from build123d import *

# Parameters (mm, degrees)
BOSS_EXTRUDE2_DEPTH                                 = 22
SKETCH6_R                                           = 35
CUT_EXTRUDE2_DEPTH                                  = 18
CHAMFER2_SIZE                                       = 2
CIRPATTERN2_COUNT                                   = 6
M8X1_0_TAPPED_HOLE1_D                               = 7
M8X1_0_TAPPED_HOLE1_DEPTH                           = 15
M8X1_0_TAPPED_HOLE1_CSINK_D                         = 8.05
M8X1_0_TAPPED_HOLE1_CSINK_ANGLE                     = 90
M8X1_0_TAPPED_HOLE1_TIP                             = 2.103012167
CSK_FOR_M8_COUNTERSUNK_FLAT_HEAD_SCREW1_D           = 6
CSK_FOR_M8_COUNTERSUNK_FLAT_HEAD_SCREW1_DEPTH       = 20
CSK_FOR_M8_COUNTERSUNK_FLAT_HEAD_SCREW1_CSINK_D     = 8
CSK_FOR_M8_COUNTERSUNK_FLAT_HEAD_SCREW1_CSINK_ANGLE = 90
CSK_FOR_M8_COUNTERSUNK_FLAT_HEAD_SCREW1_TIP         = 1.802581857
SKETCH15_R                                          = 14
BOSS_EXTRUDE3_DEPTH                                 = 7
FILLET1_R                                           = 4
SKETCH16_R                                          = 10
CUT_EXTRUDE3_DEPTH                                  = 30


with BuildPart() as part:
    # Sketch1 → Boss-Extrude2 (new body)
    with BuildSketch(Plane.XY):
        with BuildLine():
            Line((0, 47.5), (38, 47.5))
            Line((38, 47.5), (38, 28.5))
            ThreePointArc((38, 28.5), (47.349517724, -3.777985082), (33, -34.165040612))
            Line((33, -34.165040612), (33, -45.5))
            ThreePointArc((33, -45.5), (34.171572875, -48.328427125), (37, -49.5))
            Line((37, -49.5), (50, -49.5))
            Line((50, -49.5), (50, -59.5))
            Line((50, -59.5), (-50, -59.5))
            Line((-50, -59.5), (-50, -49.5))
            Line((-50, -49.5), (-37, -49.5))
            ThreePointArc((-37, -49.5), (-34.171572875, -48.328427125), (-33, -45.5))
            Line((-33, -45.5), (-33, -34.165040612))
            ThreePointArc((-33, -34.165040612), (-44.040262426, 17.796215482), (0, 47.5))
        make_face()
    extrude(amount=BOSS_EXTRUDE2_DEPTH)

    # Sketch6 → Cut-Extrude2 (cut)
    with BuildSketch(Plane.XY.offset(22)):
        Circle(SKETCH6_R)
    extrude(amount=-CUT_EXTRUDE2_DEPTH, mode=Mode.SUBTRACT)

    # Chamfer2
    chamfer2_edges = [part.edges().sort_by_distance(p)[0] for p in [
        (50, -54.5, 0),
        (-50, -54.5, 0),
        (-50, -54.5, 22),
        (50, -54.5, 22),
    ]]
    chamfer(chamfer2_edges, length=CHAMFER2_SIZE)

    # Sketch8 → M6 Tapped Hole2 (revolve, cut)
    with BuildSketch(Plane(origin=(0, 40, 22), x_dir=(0, -1, 0), z_dir=(1, 0, 0))):
        Polygon((0, 0), (0, 18.502151548), (2.5, 17), (2.5, 0.525), (3.025, 0), align=None)
    m6_tapped_hole2 = revolve(axis=Axis((0, 40, 28.35), (0, 0, -1)), mode=Mode.SUBTRACT)

    # CirPattern2: M6 Tapped Hole2 ×6 about axis
    cirpattern2_axis = Axis((0, 0, 0), (0, 0, 1))
    for i in range(1, CIRPATTERN2_COUNT):
        add(m6_tapped_hole2.rotate(cirpattern2_axis, i * 360 / CIRPATTERN2_COUNT), mode=Mode.SUBTRACT)

    # M8x1.0 Tapped Hole1
    with Locations(Plane(origin=(30.22, 47.5, 10.178935138), x_dir=(0, 0, 1), z_dir=(0, 1, 0))):
        with Locations((0, 0)):
            CounterSinkHole(M8X1_0_TAPPED_HOLE1_D / 2, M8X1_0_TAPPED_HOLE1_CSINK_D / 2, depth=M8X1_0_TAPPED_HOLE1_DEPTH, counter_sink_angle=M8X1_0_TAPPED_HOLE1_CSINK_ANGLE)
            with Locations((0, 0, -(M8X1_0_TAPPED_HOLE1_DEPTH + M8X1_0_TAPPED_HOLE1_TIP / 2))):  # 118° drill point
                Cone(0, M8X1_0_TAPPED_HOLE1_D / 2, M8X1_0_TAPPED_HOLE1_TIP, mode=Mode.SUBTRACT)

    # CSK for M8 Countersunk Flat Head Screw1
    with Locations(Plane(origin=(-42, -59.5, 11), x_dir=(-1, 0, 0), z_dir=(0, -1, 0))):
        with Locations((0, 0), (-84, 0)):
            CounterSinkHole(CSK_FOR_M8_COUNTERSUNK_FLAT_HEAD_SCREW1_D / 2, CSK_FOR_M8_COUNTERSUNK_FLAT_HEAD_SCREW1_CSINK_D / 2, depth=CSK_FOR_M8_COUNTERSUNK_FLAT_HEAD_SCREW1_DEPTH, counter_sink_angle=CSK_FOR_M8_COUNTERSUNK_FLAT_HEAD_SCREW1_CSINK_ANGLE)
            with Locations((0, 0, -(CSK_FOR_M8_COUNTERSUNK_FLAT_HEAD_SCREW1_DEPTH + CSK_FOR_M8_COUNTERSUNK_FLAT_HEAD_SCREW1_TIP / 2))):  # 118° drill point
                Cone(0, CSK_FOR_M8_COUNTERSUNK_FLAT_HEAD_SCREW1_D / 2, CSK_FOR_M8_COUNTERSUNK_FLAT_HEAD_SCREW1_TIP, mode=Mode.SUBTRACT)

    # Sketch15 → Boss-Extrude3 (add)
    with BuildSketch(Plane(origin=(0, 0, 0), x_dir=(-1, 0, 0), z_dir=(0, 0, -1))):
        Circle(SKETCH15_R)
    extrude(amount=BOSS_EXTRUDE3_DEPTH)

    # Fillet1
    fillet1_edges = [part.edges().sort_by_distance(p)[0] for p in [
        (14, 0, 0),
    ]]
    fillet(fillet1_edges, radius=FILLET1_R)

    # Sketch16 → Cut-Extrude3 (cut, through all)
    with BuildSketch(Plane(origin=(0, 0, -7), x_dir=(-1, 0, 0), z_dir=(0, 0, -1))):
        Circle(SKETCH16_R)
    extrude(amount=-CUT_EXTRUDE3_DEPTH, mode=Mode.SUBTRACT)


solid = part.part
Can you work these out from the model? Positions are in its coordinate system, mm. A direction names the side the tool comes from. Round coordinates to 2 decimals unless told otherwise and drop trailing zeros. Loops run counter-clockwise (first coordinate to the right, second up) from the corner with the lowest first, then second, coordinate; pieces in that order, holes last. Notation, with made-up numbers: (43.25, 43.25) - (58.25, 43.25) arc R35 ccw to (58.25, 79.25) - close; hole circle Ø7 at (52.25, -23). An arc over 180 degrees is marked (long way). Use CSV: the item, a comma, the result in double quotes. Start each with the question number.
1) Please list where these lines run through material, in increasing order: probe 1 along Y at (x, z) = (-2, 10.25); probe 2 along Z at (x, y) = (30, -7); probe 3 along Y at (x, z) = (-5.5, -1.5). Write a range as [from, to].
2) If we section it at D-D on x = -28: Write out the boundary of the cut face in (y, z).
3) For faces 1 (the cylindrical face through (34.141, -48.297, 10.846)), 2 (the flat face through (-33, -40, 11)), 3 (the cylindrical face through (-32.53, 21.34, 13.35)), 4 (the cylindrical face through (-12.932, -5.362, -5.479)), which set-ups out of +Z, -Z, +X, -X, +Y, -Y let a thin tool reach every point of the face, with its end or its side?
4) For pin 1 Ø8 at (x, z) = (-42, 11) entering from +Y; pin 2 Ø3 at (x, y) = (-34.64, 20) entering from +Z; pin 3 Ø6.5 at (x, y) = (34.64, -20) entering from -Z, each with a flat end and sliding along its axis, tell me the tip position at first contact or that it passes through.
5) If we section it at B-B on z = 18.5: Write out the boundary of the cut face in (x, y).
6) If we section it at A-A on y = 0: Write out the boundary of the cut face in (x, z).
7) If we section it at C-C on x = 42: Write out the boundary of the cut face in (y, z), plus the area to 3 significant figures.
8) We'd pull the mould along Z, two halves only. Please class faces 5 (the cylindrical face through (-45, -54, 11)), 6 (the conical face through (-34.21, 19.94, 3.76)), 7 (the flat face through (1, -59.5, 11)): released by +Z, released by -Z, zero draft, split by the parting line, or undercut.
Geometry results:
1,probe 1,"y = [-59.5, -41.5], [-38.5, -34.94], [34.94, 38.5], [41.5, 47.46]"
1,probe 2,"z = [0, 4]"
1,probe 3,"y = [-13.82, -8.35], [8.35, 13.82]"
2,outline,"(-59.5, 0) - (38.37, 0) - (38.37, 22) - (21, 22) - (21, 4) - (-21, 4) - (-21, 22) - (-59.5, 22) - close"
3,face 1,"+Z, -Z, +X"
3,face 2,"+Z, -Z, -X"
3,face 3,"+Z"
3,face 4,"-Z"
4,pin 1,"stops at y = 28.5"
4,pin 2,"stops at z = 4.4"
4,pin 3,"stops at z = 0"
5,outline,"(-50, -59.5) - (50, -59.5) - (50, -49.5) - (37, -49.5) arc R4 cw to (33, -45.5) - (33, -34.17) arc R47.5 ccw to (38, 28.5) - (38, 47.5) - (0, 47.5) arc R47.5 ccw to (-33, -34.17) - (-33, -45.5) arc R4 cw to (-37, -49.5) - (-50, -49.5) - close; hole circle Ø5 at (-34.64, -20); hole circle Ø5 at (-34.64, 20); hole circle Ø70 at (0, 0); hole circle Ø5 at (0, -40); hole circle Ø5 at (0, 40); hole circle Ø5 at (34.64, -20); hole circle Ø5 at (34.64, 20)"
6,outline,"(-47.5, 0) - (-18, 0) arc R4 cw to (-14, -4) - (-14, -7) - (-10, -7) - (-10, 4) - (-35, 4) - (-35, 22) - (-47.5, 22) - close; (10, -7) - (14, -7) - (14, -4) arc R4 cw to (18, 0) - (47.5, 0) - (47.5, 22) - (35, 22) - (35, 4) - (10, 4) - close"
7,outline,"(-59.5, 0) - (-49.5, 0) - (-49.5, 8) - (-58.5, 8) - (-59.5, 7) - close; (-59.5, 15) - (-58.5, 14) - (-49.5, 14) - (-49.5, 22) - (-59.5, 22) - close; (-22.19, 0) - (22.19, 0) - (22.19, 22) - (-22.19, 22) - close"
7,area,"1,140 mm2"
8,face 5,"undercut"
8,face 6,"released by +Z"
8,face 7,"zero draft"
